Check sheet for the modelled part. Datum: model origin and axes. Units: mm. A direction names the side the tool comes from. Round coordinates to 2 decimals unless told otherwise and drop trailing zeros. Write each loop counter-clockwise with the first axis right and the second up, starting at its lowest first coordinate (ties: lowest second). Pieces come first, ordered by that corner, then holes. Notation, with made-up numbers: (78, -38.75) -> (121, -38.75) arc R21 cw to (121, -18.75) -> close; hole circle Ø8 at (1, -14.5). An arc over 180 degrees is marked (long way). Write item = value, one per line.
from build123d import *

# Parameters (mm, degrees)
F1_DEPTH = 1
F3_D     = 10
F4_W     = 30.093235299
F4_H     = 10.0299605876
F5_DEPTH = 1
F7_D     = 5


with BuildPart() as f1:
    # F0 (on Front) → F1 (new body)
    with BuildSketch(Plane.XZ):
        Polygon((-15, -9.0614365251), (15, -9.0614365251), (0, 9.0614365251), align=None)
    extrude(amount=F1_DEPTH)

    # F3 (through all)
    with Locations(Plane.XZ.offset(1)):
        with Locations((0, 12.73057051)):
            Hole(F3_D / 2)

    # F4 (on face) → F5 (join)
    with BuildSketch(Plane(origin=(0, 0, -9.0614365251), x_dir=(1, 0, 0), z_dir=(0, 0, -1))):
        with Locations((0.0466176495, 6.0149802938)):
            Rectangle(F4_W, F4_H)
    extrude(amount=-F5_DEPTH)

    # F7 (through all)
    with Locations(Plane.XZ.offset(1)):
        with Locations((0, 3.6346598063)):
            Hole(F7_D / 2)


solid = f1.part
(1) Release check for a two-part mould opening along Z. For faces 1 (the flat face through (-7.91, -0.493, -0.495)), 2 (the cylindrical face through (0.325, -0.493, 6.113)), 3 (the flat face through (0, 0, -4)) record: pulls with the +Z half, pulls with the -Z half, needs draft (parallel to the pull), parting line crosses it, or undercut.
Worked answers:
face_1 = pulls with the +Z half
face_2 = undercut
face_3 = needs draft
(2) Access from +Z, -Z, +X, -X, +Y, -Y to the whole of each face (thin tool, end or side, straight path). Record for faces 4 (the flat face through (-14.8, -1, -8.3)), 5 (the flat face through (14.73, -1, -8.46)), 6 (the flat face through (0, -6, -8.061)), 7 (the cylindrical face through (0.01, -0.49, 7.73)).
Worked answers:
face_4 = +Z, -X, +Y
face_5 = +Z, +X, +Y
face_6 = +Z, +X, -X, -Y
face_7 = +Z, +Y, -Y
(3) Material ranges on L1, parallel to Z at x = -11, y = -9.5; L2, parallel to Y at x = -2, z = 5.75; L3, parallel to Z at x = -2, y = -0.5, recorded low to high. Write a range as [from, to].
Worked answers:
L1 = [-9.06, -8.06]
L2 = [-1, 0]
L3 = [-9.06, 2.13], [5.13, 6.65]
(4) Sectioned sample at C-C on y = -5.5. Enter the section's corners in (x, z), then the cut area to 3 significant figures.
Worked answers:
outline = (-15, -9.06) -> (15.09, -9.06) -> (15.09, -8.06) -> (-15, -8.06) -> close
area = 30.1 mm²
(5) Sectioned sample at B-B on z = 3. Enter the section's corners in (x, y), then the cut area to 3 significant figures.
Worked answers:
outline = (-5.02, -1) -> (-2.42, -1) -> (-2.42, 0) -> (-5.02, 0) -> close; (2.42, -1) -> (5.02, -1) -> (5.02, 0) -> (2.42, 0) -> close
area = 5.20 mm²
(6) Go/stop test with flat-tipped pins: P1, Ø5, axis at y = -4.5, z = 5.5, coming from the -X side; P2, Ø1.5, axis at x = 2.5, z = -4.5, coming from the -Y side; P3, Ø4, axis at x = 8, y = -4, coming from the +Z side; P4, Ø5, axis at y = -1.5, z = 2, coming from the -X side. Record where each tip stops, or that it passes through.
Worked answers:
P1 = through
P2 = -1
P3 = -8.06
P4 = -7.87
(7) Sectioned sample at D-D on x = 8.5. Enter the section's corners in (y, z), then the cut area to 3 significant figures.
Worked answers:
outline = (-11.03, -9.06) -> (0, -9.06) -> (0, -1.21) -> (-1, -1.21) -> (-1, -8.06) -> (-11.03, -8.06) -> close
area = 17.9 mm²
(8) Sectioned sample at A-A on x = 0. Enter the section's corners in (y, z), then the cut area to 3 significant figures.
Worked answers:
outline = (-11.03, -9.06) -> (0, -9.06) -> (0, 1.13) -> (-1, 1.13) -> (-1, -8.06) -> (-11.03, -8.06) -> close; (-1, 6.13) -> (0, 6.13) -> (0, 7.73) -> (-1, 7.73) -> close
area = 21.8 mm²
